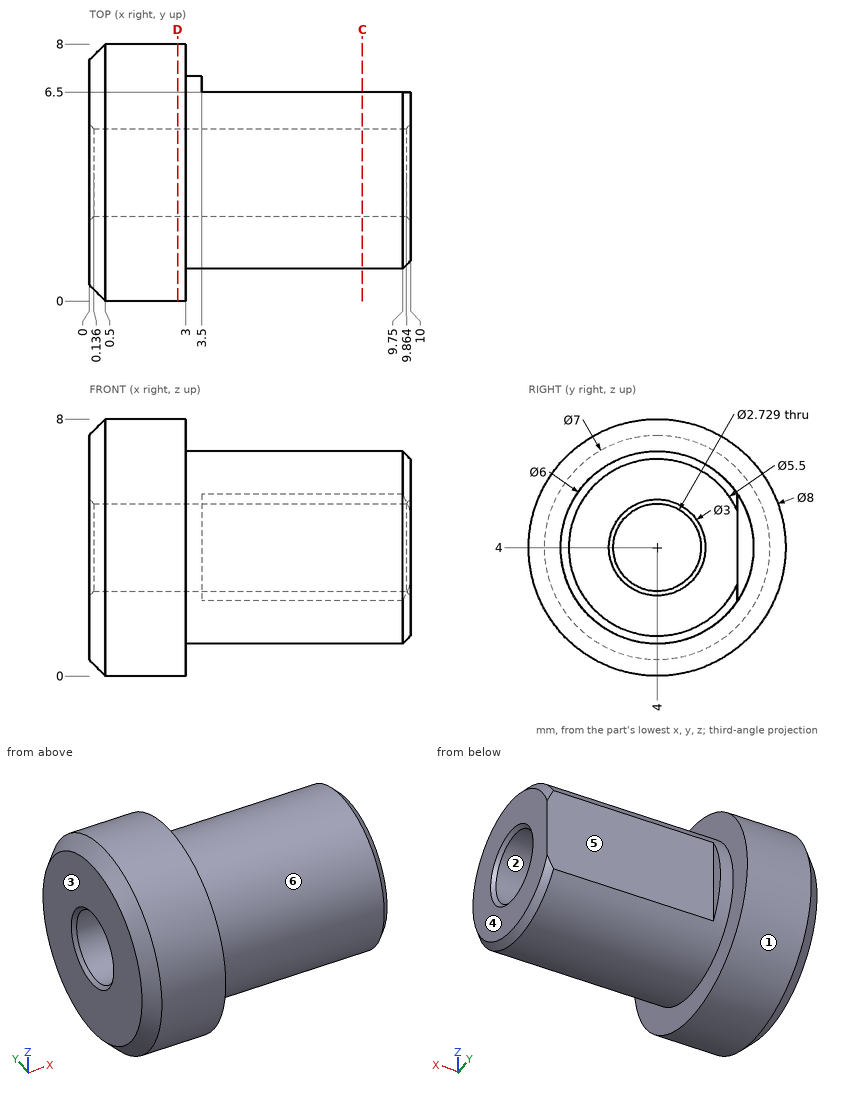
Input: dimensioned drawing with shaded views. Units: mm. Origin: part minimum x, y, z. A direction names the side the tool comes from. Give positions to 0.01 mm unless a question says otherwise; leave off trailing zeros. Write each loop counter-clockwise with the first axis right and the second up, starting at its lowest first coordinate (ties: lowest second). Pieces come first, ordered by that corner, then holes. Notation, with made-up numbers: M -35.75,-3.75 L -18.75,-3.75 A13 ccw -18.75,4.25 Z; hole C -20,-35.75 d4. An arc over 180 degrees is marked long. Return JSON: item names as keys, results as strings. Group by question number.
1) Pin query (flat end, axial travel): P1, Ø1, axis at x = 8, z = 5, coming from the +Y side; P2, Ø2.5, axis at y = 4, z = 4, coming from the +X side; P3, Ø4, axis at x = 3, y = 5.5, coming from the +Z side; P4, Ø3, axis at x = 2.5, z = 6.5, coming from the -Y side. Return the tip coordinate at first contact, or that it passes through.
2) Pull-direction query (Z, two-part tool) for the marked faces 1, 2 and 3; classes: pulls with the +Z half, pulls with the -Z half, needs draft (parallel to the pull), parting line crosses it, or undercut.
3) Material intervals for line 1 along Y through (x, z) = (3.75, 4) (1 decimal); line 2 along Y through (x, z) = (2.5, 4) (1 decimal); line 3 along X through (y, z) = (5.75, 7), sorted ascending. Write a range as [from, to].
4) Cut plane D-D, the plane x = 2.75. Output: boundary loops of the cut face in (y, z) (1 decimal).
5) Cut plane C-C, the plane x = 8.5. Output: boundary loops of the cut face in (y, z) (1 decimal), plus the area to 3 significant figures.
6) Set-up query: the marked faces 4, 5 and 6. Return all of +Z, -Z, +X, -X, +Y, -Y with unobstructed straight access to the full face (end or side cutting, diameter ignored); none if empty.
Recorded:
{
 "1": {"P1": "stops at y = 6.5", "P2": "passes through", "P3": "stops at z = 8", "P4": "stops at y = 0.13"},
 "2": {"face 1": "parting line crosses it", "face 2": "undercut", "face 3": "needs draft"},
 "3": {"line 1": "y = [1, 2.6], [5.4, 6.5]", "line 2": "y = [0, 2.6], [5.4, 8]", "line 3": "x = [0, 3]"},
 "4": {"outline": "C 4,4 d8; hole C 4,4 d2.7"},
 "5": {"outline": "M 6.5,2.3 L 6.5,5.7 A3 ccw long Z; hole C 4,4 d2.7", "area": "21.3 mm²"},
 "6": {"face 4": "+Z, -Z, +X, +Y, -Y", "face 5": "+Z, -Z, +X, +Y", "face 6": "+X"}
}
